Could you check a few things on this model? Use its own coordinates, in mm. A direction names the side the tool comes from. Round coordinates to 2 decimals unless told otherwise and drop trailing zeros. Loops run counter-clockwise (first coordinate to the right, second up) from the corner with the lowest first, then second, coordinate; pieces in that order, holes last. Notation, with made-up numbers: (-8, 81) - (-2, 81) arc R25 cw to (-2, 112) - close; hole circle Ø9 at (42, 23.5). An arc over 180 degrees is marked (long way). Use one line per item in the form item = value.
```python
from build123d import *

# Parameters (mm, degrees)
F0_W     = 151.485607028
F0_H     = 18.2879995555
F1_DEPTH = 228.6
F2_T     = -2.54
F3_R     = 10.6799813772
F3_R_2   = 11.2854145599
F3_R_3   = 10.6922207588
F3_R_4   = 10.6551247764
F8_DEPTH = 170.18


# Not quite as in the source:
# - the program builds the solid bodies; features that only make, move or delete a surface that nothing else refers to are left out


with BuildPart() as f1:
    # F0 (on Front) → F1 (new body)
    with BuildSketch(Plane.XZ):
        with Locations((0, 9.1439997777)):
            Rectangle(F0_W, F0_H)
    extrude(amount=F1_DEPTH)

    # F2
    f2_openings = [f1.faces().sort_by_distance(p)[0] for p in [
        (0, -114.3, 0),
    ]]
    offset(amount=F2_T, openings=f2_openings)

    # F3 (on face) → F8 (join)
    with BuildSketch(Plane(origin=(0, 0, 15.7479995555), x_dir=(1, 0, 0), z_dir=(0, 0, -1))):
        with Locations((-58.2167990506, 212.1407985687)):
            Circle(F3_R)
        with Locations((-56.9975972176, 18.2879958302)):
            Circle(F3_R_2)
        with Locations((60.0456036627, 18.2879958302)):
            Circle(F3_R_3)
        with Locations((60.6552027166, 210.921600461)):
            Circle(F3_R_4)
    extrude(amount=F8_DEPTH)


solid = f1.part
```
1. If we section it at A-A, the plane y = -123: Write out the boundary of the cut face in (x, z).
Solution:
outline = (-75.74, 0) - (-73.2, 0) - (-73.2, 15.75) - (73.2, 15.75) - (73.2, 0) - (75.74, 0) - (75.74, 18.29) - (-75.74, 18.29) - close
2. We'd pull the mould along Y, two halves only. Please class faces 1 (the face through (-1, 0, 9)), 2 (the face through (-59.61, -222.73, -68.15)), 3 (the face through (-58, -212, -154.432)), 4 (the face through (-1, -228.6, 9)): +Y half, -Y half, draft (parallel to the pull), parting line (faces both ways), or undercut.
Solution:
face_1 = +Y half
face_2 = undercut
face_3 = draft
face_4 = -Y half
3. On a 3-axis mill with a long thin cutter (end or side, diameter ignored), from which of +Z, -Z, +X, -X, +Y, -Y can I reach the whole of each face in a straight line? I mean faces 5 (the face through (-50.931, -27.804, -68.151)), 6 (the face through (75.743, -113, 9)). Say none if no direction works.
Solution:
face_5 = -Z
face_6 = +Z, -Z, +X, +Y, -Y
4. If we section it at B-B, the plane x = -32.5: Write out the boundary of the cut face in (y, z), plus the area to 3 significant figures.
Solution:
outline = (-228.6, 0) - (-226.06, 0) - (-226.06, 15.75) - (-2.54, 15.75) - (-2.54, 0) - (0, 0) - (0, 18.29) - (-228.6, 18.29) - close
area = 661 mm^2
5. For P1, Ø8, axis at x = 41, y = -146.5, coming from the -Z side; P2, Ø17.5, axis at x = 34.5, z = 9, coming from the +Y side; P3, Ø12, axis at x = -43.5, z = -58, coming from the +Y side, each with a flat end and sliding along its axis, tell me the tip position at first contact or that it passes through.
Solution:
P1 = 15.75
P2 = 0
P3 = -9.85
6. Please list where these lines run through material, in increasing order: line 1 along X through (y, z) = (-212, -34.5); line 2 along Z through (x, y) = (23, -78); line 3 along Y through (x, z) = (68, -36).
Solution:
line_1 = -68.9 to -47.54, 50.05 to 71.26
line_2 = 15.75 to 18.29
line_3 = -218.64 to -203.2, -25.43 to -11.14
7. If we section it at C-C, the plane z = -118: Write out the boundary of the cut face in (x, y).
Solution:
outline = circle Ø21.36 at (-58.22, -212.14); circle Ø22.57 at (-57, -18.29); circle Ø21.38 at (60.05, -18.29); circle Ø21.31 at (60.66, -210.92)
